The drawing under review shows one solid part. Ordinate dimensions are in mm from its lowest x, y, z. Coordinates: 2 decimals unless noted, no trailing zeros. Write each loop counter-clockwise with the first axis right and the second up, starting at its lowest first coordinate (ties: lowest second). Pieces come first, ordered by that corner, then holes. Notation, with made-up numbers: (56.25, 32.25) - (89.25, 32.25) arc R21 cw to (89.25, 61.25) - close; hole circle Ø2 at (53, 82.5). An arc over 180 degrees is marked (long way). Use a Markdown table: item, result.
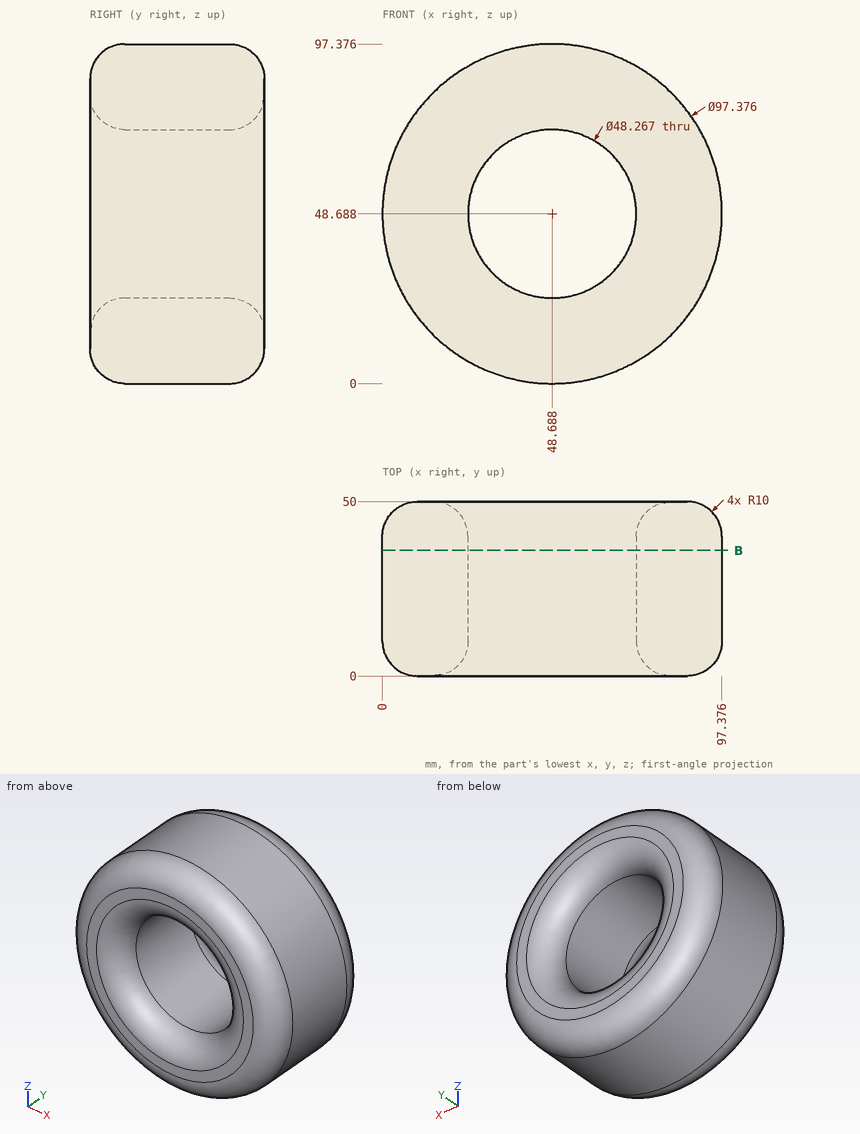
(1) Take a section at B-B on y = 36. Write out the cut boundary in (x, z), and give its area (3 significant figures).
Determined:
| item | result |
|---|---|
| outline | circle Ø97.38 at (48.69, 48.69); hole circle Ø48.27 at (48.69, 48.69) |
| area | 5,620 mm2 |
(2) For pin 1 (8 mm diameter, centred on x = 79.5, y = 28, fed in from +Z); pin 2 (2 mm diameter, centred on y = 19, z = 76.5, fed in from +X); pin 3 (8 mm diameter, centred on x = 55.5, y = 42, fed in from +Z), all flat-tipped, find the tip position at first contact; note any pin that passes through.
Determined:
| item | result |
|---|---|
| pin 1 | z = 89.33 |
| pin 2 | x = 89.33 |
| pin 3 | z = 97.27 |
(3) For L1, parallel to Z at x = 47, y = 20.5; L2, parallel to X at y = 28, z = 44.5 (1 decimal); L3, parallel to X at y = 42.5, z = 63.5 (1 decimal), list the stretches that pass through material, from the lowest coordinate up. Write a range as from..to.
Determined:
| item | result |
|---|---|
| L1 | 0.03..24.61, 72.76..97.35 |
| L2 | 0.2..24.9, 72.5..97.2 |
| L3 | 2.6..29.2, 68.1..94.7 |
